```python
from build123d import *

# Parameters (mm, degrees)
SKETCH_1_W          = 30
SKETCH_1_H          = 30
SKETCH_1_R          = 1.15
EXTRUDE_1_DEPTH     = 12
FILLET_1_R          = 28
FILLET_2_R          = 1
CUT_EXTRUDE_3_DEPTH = 22


with BuildPart() as part:
    # 草图1 → 凸台-拉伸1 (new body)
    with BuildSketch(Plane(origin=(0, 0, 0), x_dir=(1, 0, 0), z_dir=(0, 1, 0))):
        Rectangle(SKETCH_1_W, SKETCH_1_H)
        with Locations(Location((13, 13, 0), (0, 0, 270))):
            Circle(SKETCH_1_R, mode=Mode.SUBTRACT)
        with Locations(Location((13, -13, 0), (0, 0, 90))):
            Circle(SKETCH_1_R, mode=Mode.SUBTRACT)
        with Locations(Location((-13, -13, 0), (0, 0, 270))):
            Circle(SKETCH_1_R, mode=Mode.SUBTRACT)
        with Locations(Location((-13, 13, 0), (0, 0, 90))):
            Circle(SKETCH_1_R, mode=Mode.SUBTRACT)
    extrude(amount=EXTRUDE_1_DEPTH)

    # 圆角1
    fillet_1_edges = [part.edges().sort_by_distance(p)[0] for p in [
        (15, 6, 15),
    ]]
    fillet(fillet_1_edges, radius=FILLET_1_R)

    # 圆角2
    fillet_2_edges = [part.edges().sort_by_distance(p)[0] for p in [
        (-15, 6, 15),
        (-15, 6, -15),
        (15, 6, -15),
    ]]
    fillet(fillet_2_edges, radius=FILLET_2_R)

    # 草图2 → 切除-拉伸3 (cut)
    with BuildSketch(Plane(origin=(0, 0, 0), x_dir=(1, 0, 0), z_dir=(0, 1, 0))):
        with BuildLine():
            Line((8.447221814, 10.447221814), (-8.447221814, 10.447221814))
            ThreePointArc((-8.447221814, 10.447221814), (-9.861435376, 9.861435376), (-10.447221814, 8.447221814))
            Line((-10.447221814, 8.447221814), (-10.447221814, -8.447221814))
            ThreePointArc((-10.447221814, -8.447221814), (-9.784933922, -9.934005697), (-8.236695498, -10.436110617))
            ThreePointArc((-8.236695498, -10.436110617), (4.402020591, -4.402020591), (10.436110617, 8.236695498))
            ThreePointArc((10.436110617, 8.236695498), (9.934005697, 9.784933922), (8.447221814, 10.447221814))
        make_face()
    extrude(amount=CUT_EXTRUDE_3_DEPTH, mode=Mode.SUBTRACT)


solid = part.part
```
Input: part model. Units: mm. Frame: model coordinates. A direction names the side the tool comes from. Round coordinates to 2 decimals unless told otherwise and drop trailing zeros. Write each loop counter-clockwise with the first axis right and the second up, starting at its lowest first coordinate (ties: lowest second). Pieces come first, ordered by that corner, then holes. Notation, with made-up numbers: (81.5, 65.25) -> (88.5, 65.25) arc R28 cw to (88.5, 102.25) -> close; hole circle Ø10 at (79.5, 83.5). An arc over 180 degrees is marked (long way). Answer as CSV lines item,"result".
1. Section A-A (x = 7). Return the cut outline in (y, z).
Geometry says:
outline,"(0, -15) -> (12, -15) -> (12, -10.45) -> (0, -10.45) -> close; (0, 1.24) -> (12, 1.24) -> (12, 6.6) -> (0, 6.6) -> close"
2. Contact query for flat-ended pins moving along their axis: P1, Ø6, axis at y = 8.5, z = 0.5, coming from the +X side; P2, Ø3, axis at x = -13, z = -13, coming from the +Y side. Output: stop coordinate, or through.
Geometry says:
P1,"stops at x = 12.96"
P2,"stops at y = 12"
3. Mould query, pull axis X, two halves, no side actions, for faces 1 (the cylindrical face through (6.58, 6.084, 7.015)), 2 (the cylindrical face through (-14.715, 6.084, -14.699)), 3 (the cylindrical face through (-9.846, 5.916, -9.877)). Classes: +X half, -X half, draft (parallel to the pull), parting line (faces both ways), or undercut.
Geometry says:
face 1,"+X half"
face 2,"-X half"
face 3,"undercut"
4. Ray query, L1, parallel to X at y = 2, z = -14; L2, parallel to Z at x = 2, y = 7.5; L3, parallel to Z at x = -2, y = 5.5. Return the intervals inside material, ascending. Write a range as [from, to].
Geometry says:
L1,"x = [-15, -13.57], [-12.43, 12.43], [13.57, 15]"
L2,"z = [-15, -10.45], [6.47, 10.64]"
L3,"z = [-15, -10.45], [8.78, 12.75]"
5. Section C-C (y = 3). Return the cut outline in (x, z).
Geometry says:
outline,"(-15, -14) arc R1 ccw to (-14, -15) -> (14, -15) arc R1 ccw to (15, -14) -> (15, -13) arc R28 ccw to (-13, 15) -> (-14, 15) arc R1 ccw to (-15, 14) -> close; hole circle Ø2.3 at (-13, -13); hole circle Ø2.3 at (-13, 13); hole (-10.45, -8.45) arc R2 ccw to (-8.45, -10.45) -> (8.45, -10.45) arc R2 ccw to (10.44, -8.24) arc R21 ccw to (-8.24, 10.44) arc R2 ccw to (-10.45, 8.45) -> close; hole circle Ø2.3 at (13, -13)"
6. Section B-B (z = -4.5). Return the cut outline in (x, y).
Geometry says:
outline,"(-15, 0) -> (-10.45, 0) -> (-10.45, 12) -> (-15, 12) -> close; (9.69, 0) -> (13.68, 0) -> (13.68, 12) -> (9.69, 12) -> close"
7. Section D-D (z = 11). Return the cut outline in (x, y).
Geometry says:
outline,"(-15, 0) -> (1.42, 0) -> (1.42, 12) -> (-15, 12) -> close"
8. Reachability of faces 4 (the cylindrical face through (-9.8, 5.92, 9.92)), 5 (the flat face through (6, 12, 3)) from +Z, -Z, +X, -X, +Y, -Y: full face, straight path, thin tool, end or side. Return the list, or none.
Geometry says:
face 4,"+Y, -Y"
face 5,"+Z, -Z, +X, -X, +Y"
